Autodesk Inventor part; units mm, degrees
ref_plane "YZ Plane" through (0, 0, 0) normal (1, 0, 0) x (0, 1, 0)
ref_plane "XZ Plane" through (0, 0, 0) normal (0, 1, 0) x (-1, 0, 0)
ref_plane "XY Plane" through (0, 0, 0) normal (0, 0, 1) x (1, 0, 0)
sketch "Sketch1" plane through (0, 0, 0) normal (0, 1, 0) x (-1, 0, 0)
  line L0 (48.2977, 71.5211) -> (-16.7023, 71.5211)
  line L1 (-16.7023, 71.5211) -> (-16.7023, -8.4789)
  line L2 (-16.7023, -8.4789) -> (48.2977, -8.4789)
  line L3 (48.2977, -8.4789) -> (48.2977, 71.5211)
  arc A0 (22.2975, -8.4789) -> (-2.7023, -8.4789) centre (9.7976, -8.4281) ccw
  line L4 (-16.7023, -8.4789) -> (-13.7023, -8.4789)
  line L5 (-13.7023, -8.4789) -> (-13.7023, 71.5211)
  line L6 (-13.7023, 71.5211) -> (-16.7023, 71.5211)
  line L7 (-16.7023, 71.5211) -> (-16.7023, -8.4789)
  line L8 (48.2977, -8.4789) -> (40.7977, -8.4789)
  line L9 (40.7977, -8.4789) -> (40.7977, 71.5211)
  line L10 (40.7977, 71.5211) -> (48.2977, 71.5211)
  line L11 (48.2977, 71.5211) -> (48.2977, -8.4789)
  line L12 (-13.7023, -8.4789) -> (40.7977, -8.4789)
  line L13 (40.7977, -8.4789) -> (40.7977, 9.0211)
  line L14 (40.7977, 9.0211) -> (-13.7023, 9.0211)
  line L15 (-13.7023, 9.0211) -> (-13.7023, -8.4789)
  line L16 (-13.7023, 71.5211) -> (40.7977, 71.5211)
  line L17 (40.7977, 71.5211) -> (40.7977, 64.0211)
  line L18 (40.7977, 64.0211) -> (-13.7023, 64.0211)
  line L19 (-13.7023, 64.0211) -> (-13.7023, 71.5211)
  line L20 (-16.7023, 61.5211) -> (-6.7023, 71.5211)
  line L21 (-16.7023, 61.5211) -> (-16.7023, 71.5211)
  line L22 (-6.7023, 71.5211) -> (-13.7023, 64.5211)
  line L23 (-13.7023, 64.0211) -> (-13.7023, 64.5211)
  line L24 (-6.7023, 71.5211) -> (40.7977, 71.5211)
  line L25 (40.7977, 64.0211) -> (-13.7023, 64.0211)
  line L26 (-13.7023, 64.5211) -> (-13.7023, 64.0211)
  line L27 (-13.7023, 64.5211) -> (-6.7023, 71.5211)
  line L28 (-13.7023, 54.0211) -> (-3.7023, 64.0211)
  point P0 (0, 0)
  dimension "d0" = 80
  dimension "d1" = 65
  dimension "d3" = 14
  dimension "d4" = 12.5
  dimension "d5" = 7.5
  dimension "d6" = 3
  dimension "d7" = 17.5
  dimension "d8" = 7.5
  dimension "d9" = 10
  dimension "d10" = 10
  dimension "d48" = 10
  dimension "d49" = 10
extrude "Extrusion1" add sketch "Sketch1" along normal blind 100 contours L3 L2 L9 L0 | L9 L18 L5 L20 L0 | L2 A0 L5 L14 L9 | L5 L2 L1 L20
sketch "Sketch2" plane through (-22.2975, 0, -8.4789) normal (0, 0, -1) x (-1, 0, 0)
  line L0 (18.5002, 0) -> (18.5002, 100)
  line L1 (18.5002, 100) -> (-35.9998, 100)
  line L2 (-35.9998, 100) -> (-35.9998, 6.5)
  line L3 (-35.9998, 6.5) -> (18.5002, 6.5)
  line L4 (18.5002, 6.5) -> (18.5002, 100)
  point P0 (-22.2975, 0)
  dimension "d13" = 93.5
  dimension "d14" = 54.5
extrude "Extrusion2" cut sketch "Sketch2" against normal blind 30
sketch "Sketch3" plane through (-40.7977, 0, 9.0211) normal (0, 0, 1) x (1, 0, 0)
  line L0 (54.5, 6.5) -> (0, 6.5)
  line L1 (26.0002, 6.5) -> (36, 6.5)
  line L2 (18.5002, 6.5) -> (18.5002, 0)
  line L3 (43.5, 0) -> (43.5, 6.5)
  line L4 (0, 0) -> (54.5, 0)
  line L5 (36, 0) -> (26.0002, 0)
  line L6 (26.0002, 0) -> (26.0002, 3)
  line L7 (26.0002, 3) -> (36, 3)
  line L8 (36, 3) -> (36, 0)
  point P0 (40.7977, 0)
  dimension "d43" = 7.5
  dimension "d44" = 7.5
  dimension "d45" = 3
sketch "Sketch4" plane through (16.7023, 0, 61.5211) normal (1, 0, 0) x (0, 0, -1)
  line L0 (70, 100) -> (70, 6.5)
  line L1 (70, 84) -> (36, 84)
  line L2 (36, 84) -> (36, 16)
  line L3 (36, 16) -> (70, 16)
  line L4 (70, 16) -> (70, 84)
  line L5 (0, 0) -> (70, 0)
  line L6 (0, 100) -> (70, 100)
  point P0 (61.5211, 0)
  dimension "d22" = 34
  dimension "d23" = 16
  dimension "d24" = 16
  dimension "d25" = 68
extrude "Extrusion4" cut sketch "Sketch4" against normal blind 30
sketch "Sketch5" plane through (0, 0, 0) normal (0, -1, 0) x (1, 0, 0)
  line L0 (-40.7977, -8.4789) -> (-22.2975, -8.4789)
  arc A0 (-37.2975, -8.4789) -> (-34.2975, -8.4789) centre (-35.7975, -8.4789) ccw
  arc A1 (-34.2975, -8.4789) -> (-37.2975, -8.4789) centre (-35.7975, -8.4789) ccw
  point P0 (0, 0)
  dimension "d28" = 15
  dimension "d29" = 1.5
  dimension "d30" = 0
  dimension "d31" = 1.5
extrude "Extrusion5" cut sketch "Sketch5" against normal blind 30 contours A1 L0
sketch "Sketch7" plane through (-48.2977, 0, 71.5211) normal (0, 0, 1) x (1, 0, 0)
  line L0 (0, 100) -> (55, 100)
  line L1 (0, 100) -> (40, 100)
  line L2 (40, 100) -> (0, 50)
  line L3 (0, 50) -> (0, 100)
  line L4 (65, 100) -> (65, 0)
  point P0 (48.2977, 0)
  dimension "d39" = 40
  dimension "d40" = 25
  dimension "d41" = 50
extrude "Extrusion6" cut sketch "Sketch3" against normal blind 30 contours L4 L6 L7 L8
sketch "Sketch8" plane through (0, 100, 0) normal (0, 1, 0) x (1, 0, 0)
  line L0 (13.7023, 8.4789) -> (13.7023, -64.0211)
  line L1 (13.7023, -54.0211) -> (3.7023, -64.0211)
  line L2 (3.7023, -64.0211) -> (13.7023, -64.0211)
  line L3 (13.7023, -64.0211) -> (13.7023, -54.0211)
  point P0 (0, 0)
  dimension "d50" = 10
  dimension "d51" = 10
extrude "Extrusion7" add sketch "Sketch8" against normal up to surface (100 mm away)
extrude "Extrusion8" cut sketch "Sketch7" against normal blind 30
sketch "Sketch9" plane through (13.7023, 0, 9.0211) normal (-1, 0, 0) x (0, 0, 1)
  line L0 (32.5, 59.375) -> (55, 59.375)
  line L1 (45, 0) -> (45, 100)
  line L2 (45, 59.375) -> (25, 59.375)
  line L3 (25, 59.375) -> (25, 44.375)
  line L4 (25, 44.375) -> (45, 44.375)
  line L5 (45, 44.375) -> (45, 59.375)
  point P0 (-9.0211, 0)
  dimension "d56" = 15
  dimension "d57" = 20
extrude "Extrusion9" add sketch "Sketch9" along normal up to next
sketch "Sketch10" plane through (-40.7977, 44.375, 54.0211) normal (0, 0, 1) x (1, 0, 0)
  line L0 (54.5, 15) -> (0, 15)
  line L1 (55.1529, 0) -> (0.519, 0)
  line L2 (0.519, 0) -> (0.519, 15)
  line L3 (0.519, 15) -> (55.1529, 15)
  line L4 (55.1529, 15) -> (55.1529, 0)
  line L5 (54.5, 0) -> (0, 0)
  line L6 (0, 15) -> (27.836, 15)
  line L7 (27.836, 15) -> (27.836, 0)
  line L8 (27.836, 0) -> (0, 0)
  line L9 (0, 0) -> (0, 15)
  point P0 (40.7977, -44.375)
extrude "Extrusion10" add sketch "Sketch10" along normal up to next
sketch "Sketch11" plane through (13.7023, 0, 9.0211) normal (-1, 0, 0) x (0, 0, 1)
  line L0 (-17.5, 84) -> (-17.5, 100)
  line L1 (-17.5, 90) -> (12.5, 90)
  line L2 (12.5, 90) -> (12.5, 93.5)
  line L3 (12.5, 93.5) -> (-17.5, 93.5)
  line L4 (-17.5, 93.5) -> (-17.5, 90)
  line L5 (-17.5, 100) -> (45, 100)
  point P0 (-9.0211, 0)
  dimension "d62" = 3.5
  dimension "d63" = 30
  dimension "d64" = 10
extrude "Extrusion11" add sketch "Sketch11" along normal up to next
equation "\"d8\" = d5"
equation "\"d49\" = d48"
equation "\"d44\" = d43"
equation "\"d24\" = d23"
equation "\"d31\" = d29"
properties part number "Base"
Input: part model. Units: mm. Frame: model coordinates. A direction names the side the tool comes from. Give positions to 0.01 mm unless a question says otherwise; leave off trailing zeros. Order: outer loops, then holes, each group sorted by start corner. A loop starts at its lowest first (then second) coordinate and runs counter-clockwise, first axis right, second up.
Q1. Section B-B on y = 20.5. Output: boundary loops of the cut face in (x, z).
Checked values:
outline: (-48.3, -8.48) - (-40.8, -8.48) - (-40.8, 64.02) - (3.7, 64.02) - (13.7, 54.02) - (13.7, 25.52) - (16.7, 25.52) - (16.7, 61.52) - (6.7, 71.52) - (-48.3, 71.52) - close
Q2. Draft query along Z for faces 1 (the flat face through (-13, 93.5, 7)), 2 (the flat face through (-13, 52, 34.021)), 3 (the flat face through (-13, 92, 21.521)). Return one class per face: +Z half, -Z half, draft (parallel to the pull), parting line (faces both ways), or undercut.
Checked values:
face 1: draft
face 2: -Z half
face 3: undercut
Q3. Set-up query: faces 4 (the flat face through (-13.9, 3.2, 9.021)), 5 (the flat face through (-14.798, 1, 6)), 6 (the flat face through (15, 84, 8)), 7 (the flat face through (-14, 59.375, 49)). Return all of +Z, -Z, +X, -X, +Y, -Y with unobstructed straight access to the full face (end or side cutting, diameter ignored); none if empty.
Checked values:
face 4: -Y
face 5: -Z, -Y
face 6: -Z, +X
face 7: -Z, +Y
Q4. Contact query for flat-ended pins moving along their axis: pin 1 Ø8 at (x, y) = (-34.5, 85) entering from +Z; pin 2 Ø2.5 at (x, y) = (15, 50.5) entering from -Z; pin 3 Ø1.5 at (x, z) = (-32.5, 48) entering from -Y (3 decimals); pin 4 Ø15 at (x, z) = (-9, -0.5) entering from -Y. Output: stop coordinate, or through.
Checked values:
pin 1: passes through
pin 2: stops at z = 25.52
pin 3: stops at y = 44.375
pin 4: stops at y = 0
Q5. Section A-A on x = -26.5. Output: boundary loops of the cut face in (y, z) (3 decimals).
Checked values:
outline: (0, -8.479) - (6.5, -8.479) - (6.5, 9.021) - (0, 9.021) - close; (0, 64.021) - (44.375, 64.021) - (44.375, 34.021) - (59.375, 34.021) - (59.375, 64.021) - (77.247, 64.021) - (77.247, 71.521) - (0, 71.521) - close; (90, -8.479) - (93.5, -8.479) - (93.5, 21.521) - (90, 21.521) - close
Q6. Section D-D on x = -2.5. Output: boundary loops of the cut face in (y, z) (3 decimals), and give its area (3 significant figures).
Checked values:
outline: (0, 1.721) - (6.5, 1.721) - (6.5, 9.021) - (0, 9.021) - close; (0, 64.021) - (44.375, 64.021) - (44.375, 34.021) - (59.375, 34.021) - (59.375, 64.021) - (100, 64.021) - (100, 71.521) - (0, 71.521) - close; (90, -8.479) - (93.5, -8.479) - (93.5, 21.521) - (90, 21.521) - close
area: 1,350 mm2
Q7. Ray query, probe 1 along X at (y, z) = (80.5, 26.5); probe 2 along Z at (x, y) = (-12.5, 91); probe 3 along Y at (x, z) = (3.5, 2). Return the intervals inside material, ascending.
Checked values:
probe 1: x = -48.3 to -40.8, 13.7 to 16.7
probe 2: z = -8.48 to 21.52, 64.02 to 71.52
probe 3: y = 0 to 6.5, 90 to 93.5
Q8. Section C-C on z = 43. Output: boundary loops of the cut face in (x, y) (3 decimals).
Checked values:
outline: (-48.298, 0) - (-40.798, 0) - (-40.798, 44.375) - (13.702, 44.375) - (13.702, 0) - (16.702, 0) - (16.702, 100) - (13.702, 100) - (13.702, 59.375) - (-40.798, 59.375) - (-48.298, 50) - close
